Geometry: see drawing. Coordinates: mm, zero at the bounding-box minimum. A direction names the side the tool comes from. Give positions to 0.01 mm unless a question says otherwise; leave off trailing zeros. Order: outer loops, then holes, each group sorted by start corner. A loop starts at its lowest first (then second) coordinate and runs counter-clockwise, first axis right, second up. Notation, with made-up numbers: (59, 71) - (91, 71) arc R23 ccw to (91, 95) - close; hole circle Ø5 at (64.25, 39). An arc over 180 degrees is marked (long way). One line per question, with ' | ' between items. Start each with the question number.
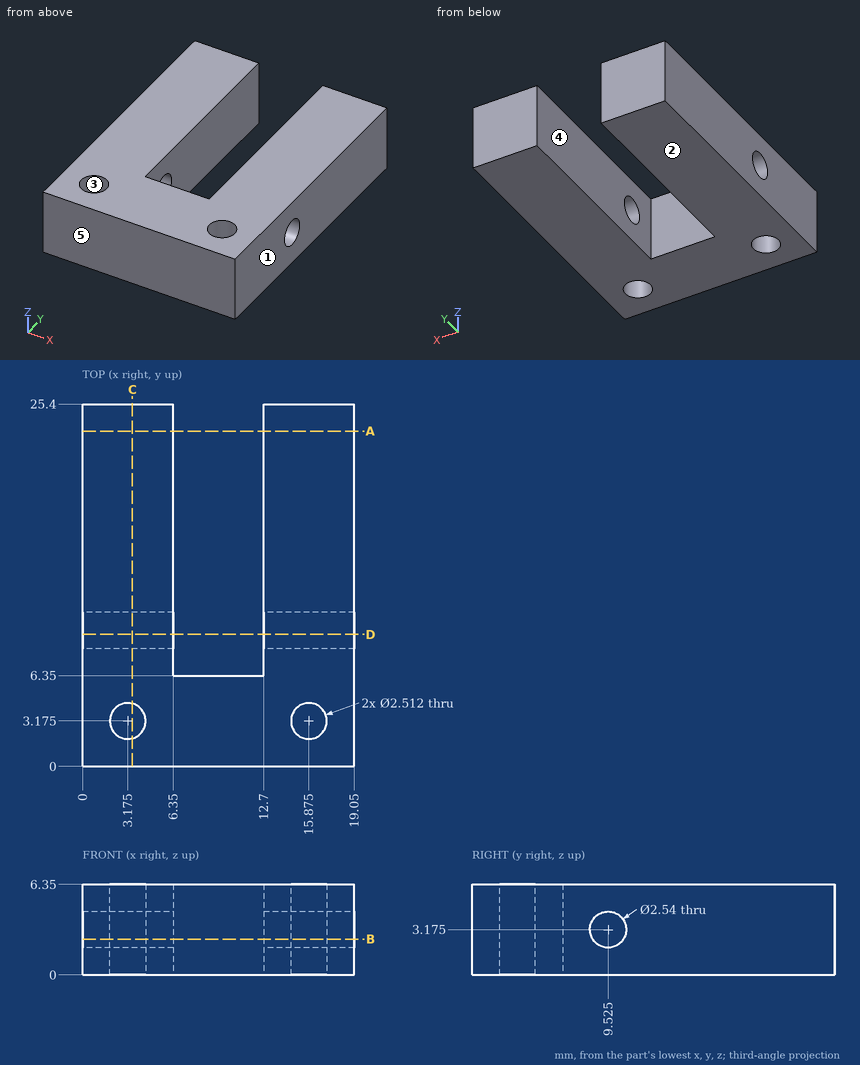
(1) Contact query for flat-ended pins moving along their axis: P1, Ø2, axis at x = 6, z = 5.5, coming from the -Y side; P2, Ø3, axis at x = 8.5, z = 3, coming from the +Y side. Output: stop coordinate, or through.
(2) Pull-direction query (X, two-part tool) for the marked faces 1, 2 and 3; classes: +X half, -X half, draft (parallel to the pull), parting line (faces both ways), or undercut.
(3) Access query for the marked faces 4 and 5. Directions: +Z, -Z, +X, -X, +Y, -Y. A direction counts if a zero-diameter tool reaches every point of the face in a straight line with its end or side. Return the directions, or none.
(4) Cut plane A-A, the plane y = 23.5. Return the cut outline in (x, z).
(5) Cut plane D-D, the plane y = 9.25. Return the cut outline in (x, z).
(6) Material intervals for line 1 along Y through (x, z) = (15.25, 2.25) (1 decimal); line 2 along Y through (x, z) = (3, 3.5); line 3 along X through (y, z) = (12, 1.5), sorted ascending. Write a range as from..to.
(7) Cut plane B-B, the plane z = 2.5. Return the cut outline in (x, y) (3 decimals).
(8) Cut plane C-C, the plane x = 3.5. Return the cut outline in (y, z) (3 decimals), plus the area to 3 significant figures.
Results are:
1) P1: y = 0 | P2: y = 6.35
2) face 1: +X half | face 2: draft | face 3: undercut
3) face 4: +Z, -Z, +Y | face 5: +Z, -Z, +X, -X, -Y
4) outline: (0, 0) - (6.35, 0) - (6.35, 6.35) - (0, 6.35) - close; (12.7, 0) - (19.05, 0) - (19.05, 6.35) - (12.7, 6.35) - close
5) outline: (0, 0) - (6.35, 0) - (6.35, 1.94) - (0, 1.94) - close; (0, 4.41) - (6.35, 4.41) - (6.35, 6.35) - (0, 6.35) - close; (12.7, 0) - (19.05, 0) - (19.05, 1.94) - (12.7, 1.94) - close; (12.7, 4.41) - (19.05, 4.41) - (19.05, 6.35) - (12.7, 6.35) - close
6) line 1: 0..2.1, 4.3..8.7, 10.4..25.4 | line 2: 0..1.93, 4.42..8.3, 10.75..25.4 | line 3: 0..6.35, 12.7..19.05
7) outline: (0, 0) - (19.05, 0) - (19.05, 8.449) - (12.7, 8.449) - (12.7, 6.35) - (6.35, 6.35) - (6.35, 8.449) - (0, 8.449) - close; (0, 10.601) - (6.35, 10.601) - (6.35, 25.4) - (0, 25.4) - close; (12.7, 10.601) - (19.05, 10.601) - (19.05, 25.4) - (12.7, 25.4) - close; hole circle Ø2.512 at (3.175, 3.175); hole circle Ø2.512 at (15.875, 3.175)
8) outline: (0, 0) - (1.962, 0) - (1.962, 6.35) - (0, 6.35) - close; (4.388, 0) - (25.4, 0) - (25.4, 6.35) - (4.388, 6.35) - close; hole circle Ø2.54 at (9.525, 3.175) | area: 141 mm2
